Could you check a few things on this model? Use its own coordinates, in mm. Face numbers are marked on the shaded views. A direction names the side the tool comes from. Give positions to 0.01 mm unless a question says otherwise; leave off trailing zeros. Loops run counter-clockwise (first coordinate to the right, second up) from the corner with the lowest first, then second, coordinate; pieces in that order, holes last. Notation, with made-up numbers: (-15.75, 50.25) - (32.25, 50.25) arc R14 cw to (32.25, 63.25) - close; hole circle Ø4 at (-22.5, 20.25). An arc over 180 degrees is marked (long way). Answer in a Markdown table with one row per item. Add a question column.
```python
from build123d import *

# Parameters (mm, degrees)
EXTRUDE_1_DEPTH      = 5
EXTRUDE_1_DEPTH_BACK = 10
SKETCH_1_W           = 8.621052632
SKETCH_1_H           = 25.2
SKETCH_1_W_2         = 5.2
SKETCH_1_H_2         = 15.2
EXTRUDE_2_DEPTH      = 25.2


with BuildPart() as part:
    # 草图1 → 凸台-拉伸1 (new, two sides: drawn at the far end of the back side and taken through both)
    with BuildSketch(Plane(origin=(0, 0, 0), x_dir=(1, 0, 0), z_dir=(0, 1, 0)).offset(-EXTRUDE_1_DEPTH_BACK)):
        Rectangle(SKETCH_1_W, SKETCH_1_H)
        Rectangle(SKETCH_1_W_2, SKETCH_1_H_2, mode=Mode.SUBTRACT)
    extrude(amount=EXTRUDE_1_DEPTH + EXTRUDE_1_DEPTH_BACK)

    # 草图2 → 凸台-拉伸2 (add)
    with BuildSketch(Plane.XY.offset(12.6)):
        Polygon((8.640653335, -7.5), (9.837723836, -4.211075827), (7.515775018, -5.551653603), (4.310526316, 0), (4.310526316, -10), align=None)
    extrude(amount=-EXTRUDE_2_DEPTH)


solid = part.part
```
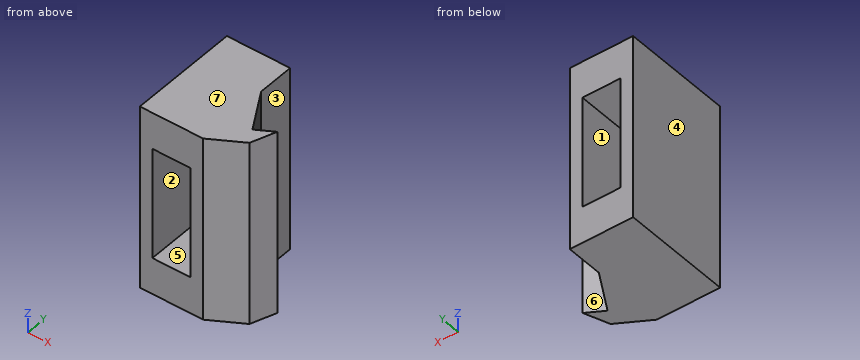
(1) Please list where these lines run through material, in increasing order: line 1 (X direction, y = 1.75, z = 7.5); line 2 (Z direction, x = -2.5, y = -5.5); line 3 (X direction, y = -2.75, z = -4.75).
(2) I want a section at A-A on z = -6. Please give me the cut outline in (x, y), then the cut area to 3 significant figures.
(3) On a 3-axis mill with a long thin cutter (end or side, diameter ignored), from which of +Z, -Z, +X, -X, +Y, -Y can I reach the whole of each face in a straight line? I mean the marked faces 5, 6 and 7. Say none if no direction works.
(4) For pin 1 Ø3 at (x, z) = (5, 8) entering from -Y; pin 2 Ø4 at (y, z) = (3.5, 1) entering from +X; pin 3 Ø2 at (x, z) = (7, 6) entering from -Y, each with a flat end and sliding along its axis, tell me the tip position at first contact or that it passes through.
(5) I want a section at C-C on z = 8. Please give me the cut outline in (x, y).
(6) I want a section at B-B on y = 2. Please give me the cut outline in (x, z).
(7) We'd pull the mould along X, two halves only. Please class the marked faces 1, 2, 3 and 4: pulls with the +X half, pulls with the -X half, needs draft (parallel to the pull), parting line crosses it, or undercut.
(8) I want a section at D-D on y = -6.5. Please give me the cut outline in (x, z), then the cut area to 3 significant figures.
Reported:
| question | item | result |
|---|---|---|
| 1 | line 1 | -4.31 to -2.6, 2.6 to 4.31 |
| 1 | line 2 | -12.6 to -7.6, 7.6 to 12.6 |
| 1 | line 3 | -4.31 to -2.6, 2.6 to 5.9 |
| 2 | outline | (-4.31, -10) - (-2.6, -10) - (-2.6, 5) - (-4.31, 5) - close; (2.6, -10) - (4.31, -10) - (8.64, -7.5) - (9.84, -4.21) - (7.52, -5.55) - (4.31, 0) - (4.31, 5) - (2.6, 5) - close |
| 2 | area | 76.0 mm² |
| 3 | face 5 | +Y, -Y |
| 3 | face 6 | +Z, -Z, +Y |
| 3 | face 7 | +Z, +X, -X, +Y, -Y |
| 4 | pin 1 | y = -10 |
| 4 | pin 2 | x = 4.31 |
| 4 | pin 3 | y = -9.02 |
| 5 | outline | (-4.31, -10) - (4.31, -10) - (8.64, -7.5) - (9.84, -4.21) - (7.52, -5.55) - (4.31, 0) - (4.31, 5) - (-4.31, 5) - close |
| 6 | outline | (-4.31, -12.6) - (4.31, -12.6) - (4.31, 12.6) - (-4.31, 12.6) - close; hole (-2.6, -7.6) - (2.6, -7.6) - (2.6, 7.6) - (-2.6, 7.6) - close |
| 7 | face 1 | undercut |
| 7 | face 2 | undercut |
| 7 | face 3 | pulls with the +X half |
| 7 | face 4 | pulls with the -X half |
| 8 | outline | (-4.31, -12.6) - (9, -12.6) - (9, 12.6) - (-4.31, 12.6) - close; hole (-2.6, -7.6) - (2.6, -7.6) - (2.6, 7.6) - (-2.6, 7.6) - close |
| 8 | area | 257 mm² |
